Autodesk Inventor part; units mm, degrees
ref_plane "YZ Plane" through (0, 0, 0) normal (1, 0, 0) x (0, 1, 0)
ref_plane "XZ Plane" through (0, 0, 0) normal (0, 1, 0) x (-1, 0, 0)
ref_plane "XY Plane" through (0, 0, 0) normal (0, 0, 1) x (1, 0, 0)
sketch "Sketch1" plane through (0, 0, 0) normal (0, 1, 0) x (-1, 0, 0)
  line L0 (-10.5, 0) -> (10.5, 0)
  line L1 (-10.5, 1.5) -> (-10.5, 10)
  line L2 (-10.5, 10) -> (-8.25, 10)
  line L3 (-8.25, 10) -> (-8.25, 5)
  line L4 (-8.25, 5) -> (-3.75, 5)
  line L5 (-3.75, 5) -> (-3.75, 10)
  line L6 (-3.75, 10) -> (-1.5, 10)
  line L7 (-1.5, 10) -> (-1.5, 4.5)
  line L8 (-1.5, 4.5) -> (10.5, 4.5)
  line L9 (10.5, 4.5) -> (10.5, 1.5)
  line L10 (10.5, 1.5) -> (-10.5, 1.5)
  line L11 (-10.5, 1.5) -> (-10.5, 0) construction
  line L12 (10.5, 1.5) -> (10.5, 0) construction
  line L13 (-8.25, 10) -> (-3.75, 10) construction
  line L14 (-6, 5) -> (-6, 1.5) construction
  line L15 (4.5, 4) -> (4.5, 1.5) construction
  point P0 (0, 0)
  point P1 (0, 0)
  dimension "d0" = 21
  dimension "d1" = 3
  dimension "d2" = 20
  dimension "d3" = 10
  dimension "d4" = 9
  dimension "d5" = 4.5
  dimension "d6" = 16.5
  dimension "d7" = 12
  dimension "d10" = 6
revolve "Revolution1" add sketch "Sketch1" angle 360 about axis through (10.5, 0, 0) along (-1, 0, 0)
sketch "Sketch2" plane through (0, 0, 0) normal (0, 0, 1) x (1, 0, 0)
  circle A0 centre (-4.5, 0) radius 1.5
  line L0 (-3.5, 4) -> (-3.5, -4)
  line L1 (-5.5, 4) -> (-5.5, -4)
  line L2 (-3.5, 0) -> (-5.5, 0) construction
  line L3 (1.5, 4.5) -> (1.5, -4.5) construction
  point P0 (0, 0)
  dimension "d12" = 3
extrude "Extrusion1" cut sketch "Sketch2" along normal through all both and the other way through all
thread "Thread1"
equation "\"d13\" = d12"
properties part number "slider-2" material "Brass, Soft Yellow"
Can you work these out from the model? Positions are in its coordinate system, mm. A direction names the side the tool comes from. Coordinates: 2 decimals unless noted, no trailing zeros. Write each loop counter-clockwise with the first axis right and the second up, starting at its lowest first coordinate (ties: lowest second). Pieces come first, ordered by that corner, then holes. Notation, with made-up numbers: (29, 59) -> (44, 59) arc R20 ccw to (44, 66) -> close; hole circle Ø10 at (70, 44). An arc over 180 degrees is marked (long way). Write item = value, one per line.
(1) Imagine slicing it at C-C (z = -7.75). Please give me the cut outline in (x, y).
Verdict:
outline = (1.5, -6.32) -> (3.75, -6.32) -> (3.75, 6.32) -> (1.5, 6.32) -> close; (8.25, -6.32) -> (10.5, -6.32) -> (10.5, 6.32) -> (8.25, 6.32) -> close
(2) On a 3-axis mill with a long thin cutter (end or side, diameter ignored), from which of +Z, -Z, +X, -X, +Y, -Y can I reach the whole of each face in a straight line? I mean faces 1 (the face through (8.25, 5, 2)), 2 (the face through (-6, 0, 3)), 3 (the face through (-4.58, -1.72, 4.16)). Say none if no direction works.
Verdict:
face_1 = none
face_2 = +Z, -Z
face_3 = -X
(3) For pin 1 (2.5 mm diameter, centred on x = -4.5, y = 0, fed in from -Z); pin 2 (8 mm diameter, centred on x = 4.5, y = -6, fed in from -Z); pin 3 (1.5 mm diameter, centred on x = -5.5, z = 3.5, fed in from -Y); pin 4 (3 mm diameter, centred on x = 1.5, z = -3, fed in from -Y), each with a flat end and sliding along its axis, tell me the tip position at first contact or that it passes through.
Verdict:
pin_1 = through
pin_2 = -9.78
pin_3 = -3.56
pin_4 = -9.89
(4) Imagine slicing it at D-D (x = 9.25). Please give me the cut outline in (y, z), and give its area (3 significant figures).
Verdict:
outline = circle Ø20 at (0, 0); hole circle Ø3 at (0, 0)
area = 307 mm^2
(5) Imagine slicing it at B-B (y = 6.25). Please give me the cut outline in (x, z).
Verdict:
outline = (1.5, -7.81) -> (3.75, -7.81) -> (3.75, 7.81) -> (1.5, 7.81) -> close; (8.25, -7.81) -> (10.5, -7.81) -> (10.5, 7.81) -> (8.25, 7.81) -> close
(6) Thinking about a two-plate mould opening in Y: for faces 4 (the face through (-8.125, -1.265, 0.806)), 5 (the face through (1.5, -2.1, 4.3)), 6 (the face through (2.61, -9.76, -2.17)), which applies, +Y half, -Y half, draft (parallel to the pull), parting line (faces both ways), or undercut?
Verdict:
face_4 = undercut
face_5 = draft
face_6 = parting line
(7) If I drill on probe 1 along Z at (x, y) = (-8.8, 0); probe 2 along Y at (x, z) = (1.75, 0), over which ranges is the centre line in solid material (lowest first)?
Verdict:
probe_1 = -4.5 to -1.5, 1.5 to 4.5
probe_2 = -10 to -1.5, 1.5 to 10
(8) Imagine slicing it at A-A (y = 0). Please give me the cut outline in (x, z), and give its area (3 significant figures).
Verdict:
outline = (-10.5, -4.5) -> (-6, -4.5) -> (-6, -1.5) -> (-10.5, -1.5) -> close; (-10.5, 1.5) -> (-6, 1.5) -> (-6, 4.5) -> (-10.5, 4.5) -> close; (-3, -4.5) -> (1.5, -4.5) -> (1.5, -10) -> (3.75, -10) -> (3.75, -5) -> (8.25, -5) -> (8.25, -10) -> (10.5, -10) -> (10.5, -1.5) -> (-3, -1.5) -> close; (-3, 1.5) -> (10.5, 1.5) -> (10.5, 10) -> (8.25, 10) -> (8.25, 5) -> (3.75, 5) -> (3.75, 10) -> (1.5, 10) -> (1.5, 4.5) -> (-3, 4.5) -> close
area = 162 mm^2
